The listing builds one solid part. Answer for the finished solid, in the listing's coordinates (mm). A direction names the side the tool comes from. Round coordinates to 2 decimals unless told otherwise and drop trailing zeros. Write each loop counter-clockwise with the first axis right and the second up, starting at its lowest first coordinate (ties: lowest second). Pieces come first, ordered by that corner, then holes.
(1) The mould has two halves that part along Y. Classify faces 4 (the face through (4, -57.5, -10)), 5 (the face through (10.48, -17.81, 1.61)), 6 (the face through (10.14, -1.25, 7.4)): +Y half, -Y half, draft (parallel to the pull), parting line (faces both ways), or undercut.
(2) For faces 1 (the face through (-2, 54.5, 2)), 2 (the face through (-5.78, -10.38, 1.65)), 3 (the face through (-2, -3, -9.5)), determine the directions among +Z, -Z, +X, -X, +Y, -Y from which every point of the face is accessible in a straight line to the end or side of a thin tool.
(3) A cutting plane is placed at C-C, the plane z = 7.5. Give the vertices of the cut face in (x, y).
(4) Find the intervals of material crossed by probe 1 along Z at (x, y) = (-7, 8.5); probe 2 along Y at (x, z) = (-5.25, 1.5); probe 3 along Y at (x, z) = (-7.75, -1.5), in increasing order.
(5) Each of these flat-tipped pins is pushed along its axis until it touches: pin 1 Ø3 at (y, z) = (17, 8) entering from -X; pin 2 Ø2 at (y, z) = (8.5, 1.5) entering from -X; pin 3 Ø6 at (x, z) = (-8, -0.5) entering from -Y; pin 4 Ø12 at (y, z) = (-39, -8.5) entering from -X. Where does it stop, or does it pass through?
(6) A cutting plane is placed at A-A, the plane x = -1. Give the vertices of the cut face in (y, z), and give its area (3 significant figures).
(7) A cutting plane is placed at D-D, the plane y = -43. Give the vertices of the cut face in (x, z).
(8) A cutting plane is placed at B-B, the plane y = 12. Give the vertices of the cut face in (x, z), and give its area (3 significant figures).
from build123d import *

# Parameters (mm, degrees)
SKETCH1_W                 = 25
SKETCH1_H                 = 115
BOSS_EXTRUDE1_DEPTH       = 14
SKETCH3_W                 = 22
SKETCH3_H                 = 112
CUT_EXTRUDE1_DEPTH        = 25
SKETCH4_W                 = 10
SKETCH4_H                 = 30
BOSS_EXTRUDE2_DEPTH       = 20
F_2_CLEARANCE_HOLE1_D     = 2.2606
F_2_CLEARANCE_HOLE1_DEPTH = 6.35
F_2_CLEARANCE_HOLE1_TIP   = 0.679152758
FILLET1_R                 = 1.5
FILLET3_R                 = 5
FILLET4_R                 = 10
FILLET5_R                 = 3
FILLET6_R                 = 3
SKETCH7_R                 = 2.5
BOSS_EXTRUDE3_DEPTH       = 8
FILLET7_R                 = 1


with BuildPart() as part:
    # Sketch1 → Boss-Extrude1 (new, symmetric)
    with BuildSketch(Plane(origin=(0, 0, 0), x_dir=(0, 0, -1), z_dir=(1, 0, 0))):
        Rectangle(SKETCH1_W, SKETCH1_H)
    extrude(amount=BOSS_EXTRUDE1_DEPTH, both=True)

    # Sketch3 → Cut-Extrude1 (cut)
    with BuildSketch(Plane(origin=(-14, 0, 0), x_dir=(0, 0, -1), z_dir=(1, 0, 0))):
        with Locations((-1.5, -1.5)):
            Rectangle(SKETCH3_W, SKETCH3_H)
    extrude(amount=CUT_EXTRUDE1_DEPTH, mode=Mode.SUBTRACT)

    # Sketch4 → Boss-Extrude2 (add)
    with BuildSketch(Plane.ZY.offset(-11)):
        with Locations((1.5, -1.5)):
            Rectangle(SKETCH4_W, SKETCH4_H)
    extrude(amount=BOSS_EXTRUDE2_DEPTH)

    # #2 Clearance Hole1
    with Locations(Plane.ZY.offset(9)):
        with Locations((1.5, 8.5), (1.5, -11.5)):
            Hole(F_2_CLEARANCE_HOLE1_D / 2, depth=F_2_CLEARANCE_HOLE1_DEPTH)
            with Locations((0, 0, -(F_2_CLEARANCE_HOLE1_DEPTH + F_2_CLEARANCE_HOLE1_TIP / 2))):  # 118° drill point
                Cone(0, F_2_CLEARANCE_HOLE1_D / 2, F_2_CLEARANCE_HOLE1_TIP, mode=Mode.SUBTRACT)

    # Fillet1
    fillet1_edges = [part.edges().sort_by_distance(p)[0] for p in [
        (-1.5, 54.5, -9.5),
        (11, 54.5, 1.5),
        (11, -1.5, -9.5),
    ]]
    fillet(fillet1_edges, radius=FILLET1_R)

    # Fillet3
    fillet3_edges = [part.edges().sort_by_distance(p)[0] for p in [
        (14, 0, -12.5),
        (0, 57.5, -12.5),
        (14, 57.5, 0),
    ]]
    fillet(fillet3_edges, radius=FILLET3_R)

    # Fillet4
    fillet4_edges = [part.edges().sort_by_distance(p)[0] for p in [
        (12.5, -57.5, 12.5),
    ]]
    fillet(fillet4_edges, radius=FILLET4_R)

    # Fillet5
    fillet5_edges = [part.edges().sort_by_distance(p)[0] for p in [
        (-14, -57.5, -11),
        (-14, 56, 12.5),
    ]]
    fillet(fillet5_edges, radius=FILLET5_R)

    # Fillet6
    fillet6_edges = [part.edges().sort_by_distance(p)[0] for p in [
        (11, -1.5, 6.5),
        (11, 13.5, 1.5),
        (11, -1.5, -3.5),
        (11, -16.5, 1.5),
    ]]
    fillet(fillet6_edges, radius=FILLET6_R)

    # Sketch7 → Boss-Extrude3 (add)
    with BuildSketch(Plane(origin=(14, 0, 0), x_dir=(0, 0, -1), z_dir=(1, 0, 0))):
        with Locations((-1.5, -43)):
            Circle(SKETCH7_R)
    extrude(amount=-BOSS_EXTRUDE3_DEPTH)

    # Fillet7
    fillet7_edges = [part.edges().sort_by_distance(p)[0] for p in [
        (6, -43, 4),
        (11, -43, 4),
    ]]
    fillet(fillet7_edges, radius=FILLET7_R)


solid = part.part
Solutions:
1. face 4: -Y half
1. face 5: undercut
1. face 6: draft
2. face 1: +Z, -X
2. face 2: -X
2. face 3: -X, -Y
3. outline: (-14, 54.5) - (9.5, 54.5) arc R1.5 cw to (11, 53) - (11, 16.5) arc R3 cw to (10.24, 14.5) - (10.24, -17.5) arc R3 cw to (11, -19.5) - (11, -56.16) - (14, -56.16) - (14, 52.5) arc R5 ccw to (9, 57.5) - (-14, 57.5) - close
4. probe 1: z = -12.5 to -9.5, -3.5 to 0.37, 2.63 to 6.5
4. probe 2: y = -16.5 to -12.63, -10.37 to 7.37, 9.63 to 13.5, 54.5 to 57.5
4. probe 3: y = -16.5 to 13.5, 54.5 to 57.5
5. pin 1: stops at x = 10.83
5. pin 2: stops at x = -2.57
5. pin 3: stops at y = -16.5
5. pin 4: stops at x = -14
6. outline: (-57.5, -12.5) - (52.5, -12.5) arc R5 ccw to (57.5, -7.5) - (57.5, 12.5) - (54.5, 12.5) - (54.5, -8) arc R1.5 cw to (53, -9.5) - (-57.5, -9.5) - close; (-16.5, -3.5) - (13.5, -3.5) - (13.5, 6.5) - (-16.5, 6.5) - close
6. area: 706 mm2
7. outline: (-14, -12.5) - (9, -12.5) arc R5 ccw to (14, -7.5) - (14, 12.5) - (11, 12.5) - (11, 5) arc R1 cw to (10, 4) - (7, 4) arc R1 ccw to (6, 3) - (6, 0) arc R1 ccw to (7, -1) - (10, -1) arc R1 cw to (11, -2) - (11, -8) arc R1.5 cw to (9.5, -9.5) - (-14, -9.5) - close
8. outline: (-14, -12.5) - (9, -12.5) arc R5 ccw to (14, -7.5) - (14, 12.5) - (11, 12.5) - (11, 9.5) arc R3 cw to (8, 6.5) - (-9, 6.5) - (-9, -3.5) - (8, -3.5) arc R3 cw to (11, -6.5) - (11, -8) arc R1.5 cw to (9.5, -9.5) - (-14, -9.5) - close
8. area: 349 mm2
